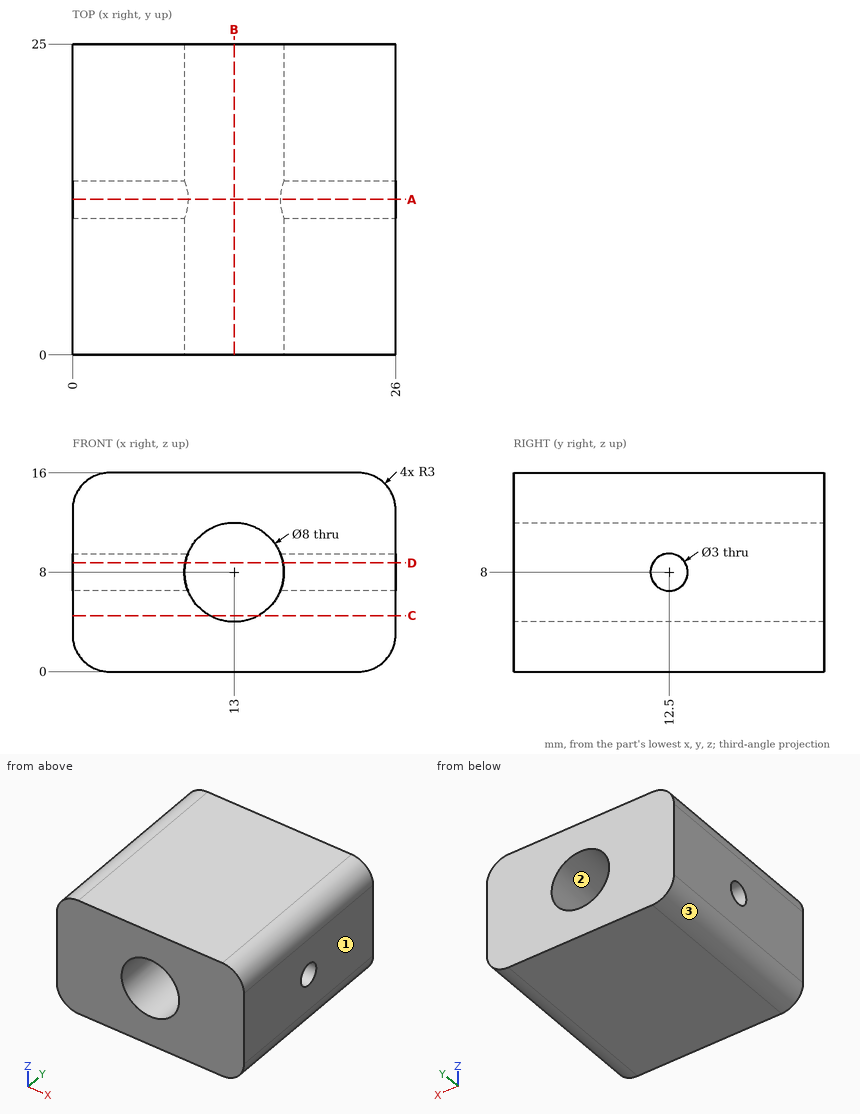
Answer from the drawing. Dimensions are ordinates in mm from the lowest x, y and z of the part. Round coordinates to 2 decimals unless told otherwise and drop trailing zeros. Write each loop counter-clockwise with the first axis right and the second up, starting at its lowest first coordinate (ties: lowest second). Pieces come first, ordered by that corner, then holes. Notation, with made-up numbers: (89.5, -8) -> (115.5, -8) arc R13 ccw to (115.5, 8) -> close; hole circle Ø10 at (-13.75, 56). An arc over 180 degrees is marked (long way). Write each question's results on one line, items separated by ' | '.
1) The part is cut by section A-A (y = 12.5). Write down the section's boundary in (x, z), and give its area (3 significant figures).
Findings:
outline: (0, 3) arc R3 ccw to (3, 0) -> (23, 0) arc R3 ccw to (26, 3) -> (26, 6.5) -> (16.71, 6.5) arc R4 cw to (9.29, 6.5) -> (0, 6.5) -> close; (0, 9.5) -> (9.29, 9.5) arc R4 cw to (16.71, 9.5) -> (26, 9.5) -> (26, 13) arc R3 ccw to (23, 16) -> (3, 16) arc R3 ccw to (0, 13) -> close | area: 303 mm²
2) The part is cut by section B-B (x = 13). Write down the section's boundary in (y, z), and give its area (3 significant figures).
Findings:
outline: (0, 0) -> (25, 0) -> (25, 4) -> (0, 4) -> close; (0, 12) -> (25, 12) -> (25, 16) -> (0, 16) -> close | area: 200 mm²
3) A flat-ended cylindrical pin translates along its axis: pin 1 (5 mm diameter, centred on x = 13, z = 8, fed in from -Y). Find the tip coordinate at first contact, or state that the pin passes through.
Findings:
pin 1: passes through
4) For a pull along X with two mould halves and no side action, classify the marked faces 1, 2 and 3 as +X half, -X half, draft (parallel to the pull), parting line (faces both ways), or undercut.
Findings:
face 1: +X half | face 2: undercut | face 3: -X half
5) The part is cut by section D-D (z = 8.75). Write down the section's boundary in (x, y).
Findings:
outline: (0, 0) -> (9.07, 0) -> (9.07, 11.2) -> (0, 11.2) -> close; (0, 13.8) -> (9.07, 13.8) -> (9.07, 25) -> (0, 25) -> close; (16.93, 0) -> (26, 0) -> (26, 11.2) -> (16.93, 11.2) -> close; (16.93, 13.8) -> (26, 13.8) -> (26, 25) -> (16.93, 25) -> close
6) The part is cut by section C-C (z = 4.5). Write down the section's boundary in (x, y), and give its area (3 significant figures).
Findings:
outline: (0, 0) -> (11.06, 0) -> (11.06, 25) -> (0, 25) -> close; (14.94, 0) -> (26, 0) -> (26, 25) -> (14.94, 25) -> close | area: 553 mm²
7) Consider line 1 along X through (y, z) = (13.5, 6.5); line 2 along X through (y, z) = (6, 8); line 3 along Z through (x, y) = (14, 20.5). Determine where each line is inside the solid, lowest interval first. Write a range as [from, to].
Findings:
line 1: x = [0, 9.29], [16.71, 26] | line 2: x = [0, 9], [17, 26] | line 3: z = [0, 4.13], [11.87, 16]
